Design review of the part built by this model. Coordinates are the model's own, in mm. A direction names the side the tool comes from. Coordinates: 2 decimals unless noted, no trailing zeros. Write each loop counter-clockwise with the first axis right and the second up, starting at its lowest first coordinate (ties: lowest second). Pieces come first, ordered by that corner, then holes. Notation, with made-up numbers: (22, -0.75) - (47, -0.75) arc R32 ccw to (47, 34.25) - close; hole circle Ø5 at (29.5, 35.25). An arc over 180 degrees is marked (long way). Answer as CSV lines item,"result". Start each with the question number.
Q1. Clearance check with flat-ended pins moving along their axes: pin 1 (0.8 mm diameter, centred on x = 175.5, y = 1.5, fed in from -Z); pin 2 (1.4 mm diameter, centred on x = 192.5, y = 1, fed in from +Z). State where each tip first meets the part, or that it passes through.
Q2. Mouldability with a two-part tool opening along X and no side actions: class faces 6 (the face through (204.579, 1, -36)), 7 (the face through (189.829, 1, -44)), 8 (the face through (127.279, 1, 27)) as pulls with the +X half, pulls with the -X half, needs draft (parallel to the pull), parting line crosses it, or undercut.
Q3. We need section A-A (z = -1). Write out the cut boundary in (x, y), plus the area to 3 significant figures.
Q4. We need section B-B (x = 179.5). Write out the cut boundary in (y, z).
Q5. Machinability: for faces 1 (the face through (129, 1, -4.4)), 2 (the face through (206, 1, 13.6)), 3 (the face through (135.829, 1, 44)), 4 (the face through (127.279, 1, -27)), 5 (the face through (198.729, 1, -44)), which of the approach directions +Z, -Z, +X, -X, +Y, -Y give a long, thin tool a straight path to every point of the face, cutting with its end or side? Answer none if there is none.
Q6. For line 1 along X through (y, z) = (1.65, -4); line 2 along Z through (x, y) = (180.5, 1.3), list the stretches that pass through material, from the lowest coordinate up. Write a range as [from, to].
from build123d import *

# Parameters (mm, degrees)
ESQUISSE1_W                    = 80
ESQUISSE1_H                    = 90
BOSS_EXTRU_1_DEPTH             = 2.7
ESQUISSE2_W                    = 2.7
ESQUISSE2_H                    = 8.8
ENL_V_MAT_EXTRU_1_DEPTH        = 2.7
R_P_TITION_LIN_AIRE1_COUNT     = 3
R_P_TITION_LIN_AIRE1_PITCH     = 18
R_P_TITION_LIN_AIRE1_COL_COUNT = 3
R_P_TITION_LIN_AIRE1_COL_PITCH = 18
SYM_TRIE1_COPY_1_SKETCH_W      = 2.7
SYM_TRIE1_COPY_1_SKETCH_H      = 8.8
SYM_TRIE1_COPY_1_DEPTH         = 2.7
SYM_TRIE1_COPY_2_SKETCH_W      = 2.7
SYM_TRIE1_COPY_2_SKETCH_H      = 8.8
SYM_TRIE1_COPY_2_DEPTH         = 2.7
SYM_TRIE1_COPY_3_SKETCH_W      = 2.7
SYM_TRIE1_COPY_3_SKETCH_H      = 8.8
SYM_TRIE1_COPY_3_DEPTH         = 2.7
SYM_TRIE1_COPY_4_SKETCH_W      = 2.7
SYM_TRIE1_COPY_4_SKETCH_H      = 8.8
SYM_TRIE1_COPY_4_DEPTH         = 2.7
ESQUISSE3_W                    = 8.9
ESQUISSE3_H                    = 2.7
ENL_V_MAT_EXTRU_2_DEPTH        = 2.7
R_P_TITION_LIN_AIRE2_COUNT     = 2
R_P_TITION_LIN_AIRE2_PITCH     = 18
R_P_TITION_LIN_AIRE2_COL_COUNT = 3
R_P_TITION_LIN_AIRE2_COL_PITCH = 18
SYM_TRIE2_COPY_1_SKETCH_W      = 8.9
SYM_TRIE2_COPY_1_SKETCH_H      = 2.7
SYM_TRIE2_COPY_1_DEPTH         = 2.7
SYM_TRIE2_COPY_2_SKETCH_W      = 8.9
SYM_TRIE2_COPY_2_SKETCH_H      = 2.7
SYM_TRIE2_COPY_2_DEPTH         = 2.7
SYM_TRIE2_COPY_3_SKETCH_W      = 8.9
SYM_TRIE2_COPY_3_SKETCH_H      = 2.7
SYM_TRIE2_COPY_3_DEPTH         = 2.7


with BuildPart() as part:
    # Esquisse1 → Boss.-Extru.1 (new body)
    with BuildSketch(Plane(origin=(0, 0, 0), x_dir=(1, 0, 0), z_dir=(0, 1, 0))):
        with Locations((167.279220614, 0)):
            Rectangle(ESQUISSE1_W, ESQUISSE1_H)
    extrude(amount=BOSS_EXTRU_1_DEPTH)

    # Esquisse2 → Enlèv. mat.-Extru.1 (cut)
    with BuildSketch(Plane(origin=(0, 0, 0), x_dir=(1, 0, 0), z_dir=(0, 1, 0))):
        with Locations((205.929220614, 0)):
            Rectangle(ESQUISSE2_W, ESQUISSE2_H)
    enl_v_mat_extru_1 = extrude(amount=ENL_V_MAT_EXTRU_1_DEPTH, mode=Mode.SUBTRACT)

    # Répétition linéaire1: Enlèv. mat.-Extru.1 ×3
    with Locations(*[(0, 0, i * R_P_TITION_LIN_AIRE1_PITCH) for i in range(1, R_P_TITION_LIN_AIRE1_COUNT)]):
        add(enl_v_mat_extru_1, mode=Mode.SUBTRACT)

    # Répétition linéaire1 col: Enlèv. mat.-Extru.1 ×3
    with Locations(*[(0, 0, -i * R_P_TITION_LIN_AIRE1_COL_PITCH) for i in range(1, R_P_TITION_LIN_AIRE1_COL_COUNT)]):
        add(enl_v_mat_extru_1, mode=Mode.SUBTRACT)

    # Symétrie1: Enlèv. mat.-Extru.1 across plane
    add(enl_v_mat_extru_1.mirror(Plane(origin=(167.279220614, 0, 0), x_dir=(0, 0, 1), z_dir=(1, 0, 0))), mode=Mode.SUBTRACT)

    # Symétrie1 copy 1 sketch → Symétrie1 copy 1 (cut)
    with BuildSketch(Plane(origin=(334.558441227, 0, 18), x_dir=(-1, 0, 0), z_dir=(0, 1, 0))):
        with Locations((205.929220614, 0)):
            Rectangle(SYM_TRIE1_COPY_1_SKETCH_W, SYM_TRIE1_COPY_1_SKETCH_H)
    extrude(amount=SYM_TRIE1_COPY_1_DEPTH, mode=Mode.SUBTRACT)

    # Symétrie1 copy 2 sketch → Symétrie1 copy 2 (cut)
    with BuildSketch(Plane(origin=(334.558441227, 0, 36), x_dir=(-1, 0, 0), z_dir=(0, 1, 0))):
        with Locations((205.929220614, 0)):
            Rectangle(SYM_TRIE1_COPY_2_SKETCH_W, SYM_TRIE1_COPY_2_SKETCH_H)
    extrude(amount=SYM_TRIE1_COPY_2_DEPTH, mode=Mode.SUBTRACT)

    # Symétrie1 copy 3 sketch → Symétrie1 copy 3 (cut)
    with BuildSketch(Plane(origin=(334.558441227, 0, -18), x_dir=(-1, 0, 0), z_dir=(0, 1, 0))):
        with Locations((205.929220614, 0)):
            Rectangle(SYM_TRIE1_COPY_3_SKETCH_W, SYM_TRIE1_COPY_3_SKETCH_H)
    extrude(amount=SYM_TRIE1_COPY_3_DEPTH, mode=Mode.SUBTRACT)

    # Symétrie1 copy 4 sketch → Symétrie1 copy 4 (cut)
    with BuildSketch(Plane(origin=(334.558441227, 0, -36), x_dir=(-1, 0, 0), z_dir=(0, 1, 0))):
        with Locations((205.929220614, 0)):
            Rectangle(SYM_TRIE1_COPY_4_SKETCH_W, SYM_TRIE1_COPY_4_SKETCH_H)
    extrude(amount=SYM_TRIE1_COPY_4_DEPTH, mode=Mode.SUBTRACT)

    # Esquisse3 → Enlèv. mat.-Extru.2 (cut)
    with BuildSketch(Plane(origin=(0, 0, 0), x_dir=(1, 0, 0), z_dir=(0, 1, 0))):
        with Locations((176.279220614, 43.65)):
            Rectangle(ESQUISSE3_W, ESQUISSE3_H)
    enl_v_mat_extru_2 = extrude(amount=ENL_V_MAT_EXTRU_2_DEPTH, mode=Mode.SUBTRACT)

    # Répétition linéaire2: Enlèv. mat.-Extru.2 ×2
    with Locations(*[(i * R_P_TITION_LIN_AIRE2_PITCH, 0, 0) for i in range(1, R_P_TITION_LIN_AIRE2_COUNT)]):
        add(enl_v_mat_extru_2, mode=Mode.SUBTRACT)

    # Répétition linéaire2 col: Enlèv. mat.-Extru.2 ×3
    with Locations(*[(-i * R_P_TITION_LIN_AIRE2_COL_PITCH, 0, 0) for i in range(1, R_P_TITION_LIN_AIRE2_COL_COUNT)]):
        add(enl_v_mat_extru_2, mode=Mode.SUBTRACT)

    # Symétrie2: Enlèv. mat.-Extru.2 across plane
    add(enl_v_mat_extru_2.mirror(Plane.XY), mode=Mode.SUBTRACT)

    # Symétrie2 copy 1 sketch → Symétrie2 copy 1 (cut)
    with BuildSketch(Plane(origin=(18, 0, 0), x_dir=(1, 0, 0), z_dir=(0, 1, 0))):
        with Locations((176.279220614, -43.65)):
            Rectangle(SYM_TRIE2_COPY_1_SKETCH_W, SYM_TRIE2_COPY_1_SKETCH_H)
    extrude(amount=SYM_TRIE2_COPY_1_DEPTH, mode=Mode.SUBTRACT)

    # Symétrie2 copy 2 sketch → Symétrie2 copy 2 (cut)
    with BuildSketch(Plane(origin=(-18, 0, 0), x_dir=(1, 0, 0), z_dir=(0, 1, 0))):
        with Locations((176.279220614, -43.65)):
            Rectangle(SYM_TRIE2_COPY_2_SKETCH_W, SYM_TRIE2_COPY_2_SKETCH_H)
    extrude(amount=SYM_TRIE2_COPY_2_DEPTH, mode=Mode.SUBTRACT)

    # Symétrie2 copy 3 sketch → Symétrie2 copy 3 (cut)
    with BuildSketch(Plane(origin=(-36, 0, 0), x_dir=(1, 0, 0), z_dir=(0, 1, 0))):
        with Locations((176.279220614, -43.65)):
            Rectangle(SYM_TRIE2_COPY_3_SKETCH_W, SYM_TRIE2_COPY_3_SKETCH_H)
    extrude(amount=SYM_TRIE2_COPY_3_DEPTH, mode=Mode.SUBTRACT)


solid = part.part
Results list:
1,pin 1,"stops at z = -42.3"
1,pin 2,"stops at z = 42.3"
2,face 6,"pulls with the +X half"
2,face 7,"undercut"
2,face 8,"pulls with the -X half"
3,outline,"(129.98, 0) - (204.58, 0) - (204.58, 2.7) - (129.98, 2.7) - close"
3,area,"201 mm2"
4,outline,"(0, -42.3) - (2.7, -42.3) - (2.7, 42.3) - (0, 42.3) - close"
5,face 1,"-X, +Y, -Y"
5,face 2,"+X, +Y, -Y"
5,face 3,"+Z, +Y, -Y"
5,face 4,"+Z, -Z, -X, +Y, -Y"
5,face 5,"-Z, +Y, -Y"
6,line 1,"x = [129.98, 204.58]"
6,line 2,"z = [-42.3, 42.3]"
